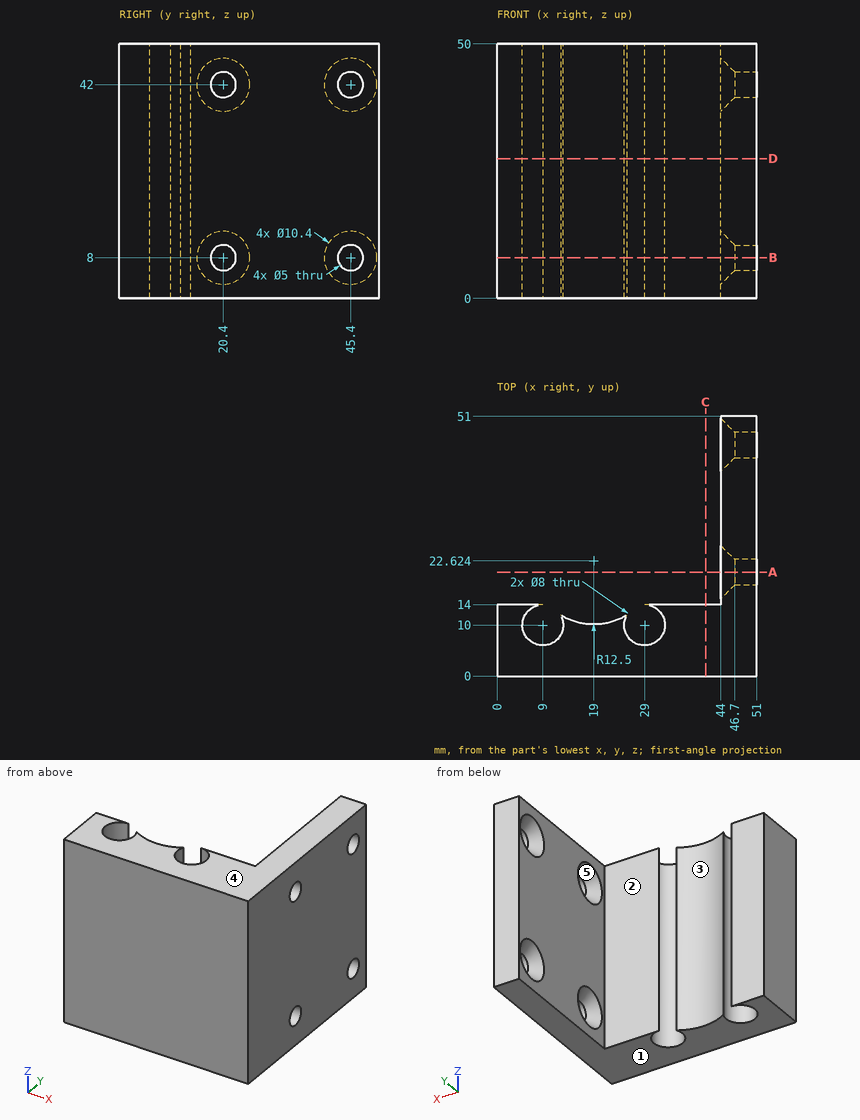
Could you check a few things on this drawing? It's one solid part, dimensions in mm from its lowest x, y, z. A direction names the side the tool comes from. Give positions to 0.01 mm unless a question says otherwise; leave off trailing zeros. Write each loop counter-clockwise with the first axis right and the second up, starting at its lowest first coordinate (ties: lowest second). Pieces come first, ordered by that corner, then holes. Notation, with made-up numbers: M 0,89 L 8,89 A19 cw 8,115 Z; hole C -11.5,58.5 d11. An arc over 180 degrees is marked long. Put each result on its own line as item: value. Start each with the question number.
Item 1: If we section it at B-B, the plane z = 8: Write out the boundary of the cut face in (x, y) (1 decimal).
Item 2: On a 3-axis mill with a long thin cutter (end or side, diameter ignored), from which of +Z, -Z, +X, -X, +Y, -Y can I reach the whole of each face in a straight line? I mean the marked faces 1 and 2. Say none if no direction works.
Item 3: If we section it at D-D, the plane z = 27.5: Write out the boundary of the cut face in (x, y) (1 decimal).
Item 4: If we section it at A-A, the plane y = 20.4: Write out the boundary of the cut face in (x, z).
Item 5: Will these pins go through, and if not, where does the flat tip stop? pin 1 (2 mm diameter, centred on x = 16, z = 36.5, fed in from -Y); pin 2 (12 mm diameter, centred on x = 32.5, z = 28.5, fed in from +Y); pin 3 (10 mm diameter, centred on y = 19.5, z = 16, fed in from -X).
Item 6: I need wall thicknesses on L1, parallel to X at y = 10, z = 31; L2, parallel to Z at x = 50.1, y = 45.4; L3, parallel to X at y = 8.5, z = 47.5. Which ranges of each line are inside material? Lowest first, please. Write a range as from..to.
Item 7: If we section it at C-C, the plane x = 41: Write out the boundary of the cut face in (y, z), then the cut area to 3 significant figures.
Item 8: Thinking about a two-plate mould opening in Z: for the marked faces 3, 4 and 5, which applies, +Z half, -Z half, draft (parallel to the pull), parting line (faces both ways), or undercut?
Values:
1. outline: M 0,0 L 51,0 L 51,17.9 L 46.7,17.9 L 44,15.2 L 44,14 L 29,14 A4 cw long 25.5,12 A12.5 cw 12.5,12 A4 cw long 9,14 L 0,14 Z; M 44,25.6 L 46.7,22.9 L 51,22.9 L 51,42.9 L 46.7,42.9 L 44,40.2 Z; M 44,50.6 L 46.7,47.9 L 51,47.9 L 51,51 L 44,51 Z
2. face 1: -Z, +X, -X, +Y, -Y
2. face 2: +Z, -Z, -X, +Y
3. outline: M 0,0 L 51,0 L 51,51 L 44,51 L 44,14 L 29,14 A4 cw long 25.5,12 A12.5 cw 12.5,12 A4 cw long 9,14 L 0,14 Z
4. outline: M 44,0 L 51,0 L 51,5.5 L 46.7,5.5 L 44,2.8 Z; M 44,13.2 L 46.7,10.5 L 51,10.5 L 51,39.5 L 46.7,39.5 L 44,36.8 Z; M 44,47.2 L 46.7,44.5 L 51,44.5 L 51,50 L 44,50 Z
5. pin 1: y = 0
5. pin 2: y = 14
5. pin 3: x = 44
6. L1: 0..5, 13..25, 33..51
6. L2: 0..5.5, 10.5..39.5, 44.5..50
6. L3: 0..5.29, 12.71..25.29, 32.71..51
7. outline: M 0,0 L 14,0 L 14,50 L 0,50 Z
7. area: 700 mm²
8. face 3: draft
8. face 4: +Z half
8. face 5: undercut
